```python
from build123d import *

# Parameters (mm, degrees)
BOSS_EXTRUDE1_DEPTH                                 = 40
CUT_EXTRUDE1_DEPTH                                  = 38
BOSS_EXTRUDE2_REACH                                 = 22
SKETCH6_W                                           = 7.999999469
SKETCH6_H                                           = 7.25
BOSS_EXTRUDE3_REACH                                 = 22
SKETCH7_W                                           = 7.999999468
SKETCH7_H                                           = 7.25
SKETCH8_W                                           = 7.999999727
SKETCH8_H                                           = 7.25
BOSS_EXTRUDE4_DEPTH                                 = 19
SKETCH9_W                                           = 7.999999728
SKETCH9_H                                           = 7.25
BOSS_EXTRUDE5_DEPTH                                 = 19
CUT_EXTRUDE4_DEPTH                                  = 0.5
BOSS_EXTRUDE6_DEPTH                                 = 0.5
CUT_EXTRUDE5_START                                  = 1.500005
CUT_EXTRUDE5_DEPTH                                  = 0.5
F_3_CLEARANCE_HOLE1_D                               = 3
F_3_CLEARANCE_HOLE1_DEPTH                           = 0.5
CBORE_FOR_4_BINDING_HEAD_MACHINE_SCREW1_D           = 3.2
CBORE_FOR_4_BINDING_HEAD_MACHINE_SCREW1_DEPTH       = 28
CBORE_FOR_4_BINDING_HEAD_MACHINE_SCREW1_CBORE_D     = 6
CBORE_FOR_4_BINDING_HEAD_MACHINE_SCREW1_CBORE_DEPTH = 19.000000001
CBORE_FOR_4_BINDING_HEAD_MACHINE_SCREW2_D           = 3.2
CBORE_FOR_4_BINDING_HEAD_MACHINE_SCREW2_DEPTH       = 25.25
CBORE_FOR_4_BINDING_HEAD_MACHINE_SCREW2_CBORE_D     = 6
CBORE_FOR_4_BINDING_HEAD_MACHINE_SCREW2_CBORE_DEPTH = 16.250000001
CHAMFER2_SIZE                                       = 0.8
FILLET1_R                                           = 1
FILLET2_R                                           = 4


with BuildPart() as part:
    # Sketch1 → Boss-Extrude1 (new body)
    with BuildSketch(Plane(origin=(19.860869514, 0, 0), x_dir=(0, 0, -1), z_dir=(1, 0, 0))):
        Polygon((0.020116779, -25.909092826), (0.020116779, 25.590907174), (-17.979883221, 25.590907174), (-27.979883221, 15.590907174), (-27.979883221, -25.909092826), align=None)
    extrude(amount=-BOSS_EXTRUDE1_DEPTH)

    # Sketch2 → Cut-Extrude1 (cut)
    with BuildSketch(Plane(origin=(-19.139130486, 0, 0), x_dir=(0, -1, 0), z_dir=(-1, 0, 0))):
        Polygon((-24.590907174, 17.565669658), (-24.590907174, -0.020116779), (24.909092826, -0.020116779), (24.909092826, 26.979883221), (-15.176693611, 26.979883221), align=None)
    extrude(amount=-CUT_EXTRUDE1_DEPTH, mode=Mode.SUBTRACT)

    # Sketch6 → Boss-Extrude2 (add, up to next)
    with BuildSketch(Plane(origin=(0, 0, 7.979883221), x_dir=(-1, 0, 0), z_dir=(0, 0, -1)), mode=Mode.PRIVATE) as boss_extrude2_sk1:
        with Locations((15.139130752, 20.965907174)):
            Rectangle(SKETCH6_W, SKETCH6_H)
    boss_extrude2_tool1 = extrude(boss_extrude2_sk1.sketch, amount=-BOSS_EXTRUDE2_REACH, mode=Mode.PRIVATE) - part.part
    add(boss_extrude2_tool1.solids().sort_by_distance((-15.139131, 20.965907, 7.979883))[0])

    # Sketch7 → Boss-Extrude3 (add, up to next)
    with BuildSketch(Plane(origin=(0, 0, 7.979883221), x_dir=(-1, 0, 0), z_dir=(0, 0, -1)), mode=Mode.PRIVATE) as boss_extrude3_sk1:
        with Locations((-14.86086978, 20.965907174)):
            Rectangle(SKETCH7_W, SKETCH7_H)
    boss_extrude3_tool1 = extrude(boss_extrude3_sk1.sketch, amount=-BOSS_EXTRUDE3_REACH, mode=Mode.PRIVATE) - part.part
    add(boss_extrude3_tool1.solids().sort_by_distance((14.86087, 20.965907, 7.979883))[0])

    # Sketch8 → Boss-Extrude4 (add)
    with BuildSketch(Plane(origin=(0, 0, 26.979883221), x_dir=(-1, 0, 0), z_dir=(0, 0, -1))):
        with Locations((-14.86086965, -21.284092826)):
            Rectangle(SKETCH8_W, SKETCH8_H)
    extrude(amount=BOSS_EXTRUDE4_DEPTH)

    # Sketch9 → Boss-Extrude5 (add)
    with BuildSketch(Plane(origin=(0, 0, 26.979883221), x_dir=(-1, 0, 0), z_dir=(0, 0, -1))):
        with Locations((15.139130622, -21.284092826)):
            Rectangle(SKETCH9_W, SKETCH9_H)
    extrude(amount=BOSS_EXTRUDE5_DEPTH)

    # Sketch10 → Cut-Extrude4 (cut)
    with BuildSketch(Plane.XY.offset(27.979883221)):
        with BuildLine():
            Line((14.150288676, -11.659092827), (2.025933023, 9.340907173))
            ThreePointArc((2.025933023, 9.340907173), (-0.139130487, 10.590907173), (-2.304193997, 9.340907173))
            Line((-2.304193997, 9.340907173), (-14.42854965, -11.659092827))
            ThreePointArc((-14.42854965, -11.659092827), (-14.42854965, -14.159092826), (-12.263486141, -15.409092826))
            Line((-12.263486141, -15.409092826), (11.985225167, -15.409092826))
            ThreePointArc((11.985225167, -15.409092826), (14.150288676, -14.159092826), (14.150288676, -11.659092827))
        make_face()
    extrude(amount=-CUT_EXTRUDE4_DEPTH, mode=Mode.SUBTRACT)

    # Sketch11 → Boss-Extrude6 (add)
    with BuildSketch(Plane.XY.offset(27.479883221)):
        with BuildLine():
            Line((-13.129511542, -12.409092827), (-1.005155889, 8.590907173))
            ThreePointArc((-1.005155889, 8.590907173), (-0.139130485, 9.090907174), (0.72689492, 8.590907173))
            Line((0.72689492, 8.590907173), (12.851250572, -12.409092827))
            ThreePointArc((12.851250572, -12.409092827), (12.851250572, -13.409092827), (11.985225169, -13.909092826))
            Line((11.985225169, -13.909092826), (-12.263486138, -13.909092826))
            ThreePointArc((-12.263486138, -13.909092826), (-13.129511542, -13.409092827), (-13.129511542, -12.409092827))
        make_face()
    extrude(amount=BOSS_EXTRUDE6_DEPTH)

    # Sketch12 → Cut-Extrude5 (cut)
    with BuildSketch(Plane.XY.offset(26.479878344).offset(CUT_EXTRUDE5_START)):
        with BuildLine():
            Line((-1.181805728, -4.919953815), (-1.557388601, 0.642194436))
            add(Edge.make_bspline(
                [(-1.557388601, 0.642194436), (-1.562255195, 0.726894151), (-1.57197876, 0.896126108), (-1.573630596, 1.150381332), (-1.563491274, 1.404367732), (-1.539477279, 1.657492298), (-1.498601615, 1.908446588), (-1.435950641, 2.155034423), (-1.347824447, 2.394209038), (-1.227947002, 2.620066875), (-1.070203444, 2.821498256), (-0.873757735, 2.98640743), (-0.644495445, 3.100925878), (-0.395458992, 3.166647074), (-0.224777297, 3.173588668), (-0.139130486, 3.177071908)],
                knots=[0, 0, 0, 0, 0.076934304, 0.153716488, 0.230489845, 0.307379808, 0.384178278, 0.460861998, 0.537777924, 0.614835636, 0.691825929, 0.768406055, 0.845421183, 0.922433493, 1, 1, 1, 1], degree=3))
            add(Edge.make_bspline(
                [(-0.139130486, 3.177071908), (-0.065510928, 3.174528216), (0.081440904, 3.169450757), (0.298073955, 3.121720242), (0.503386356, 3.037662683), (0.688981961, 2.914531923), (0.846742946, 2.757270627), (0.974882351, 2.575723676), (1.075136008, 2.378059028), (1.151690203, 2.170509138), (1.208454116, 1.957026535), (1.248786563, 1.740308946), (1.275266584, 1.522162803), (1.290343043, 1.303017743), (1.295405911, 1.083047008), (1.292059183, 0.862557831), (1.283440251, 0.71568476), (1.279127629, 0.642194436)],
                knots=[0, 0, 0, 0, 0.06668985, 0.133119456, 0.199920485, 0.266795101, 0.333669142, 0.400733876, 0.467442387, 0.534072191, 0.600968136, 0.667508068, 0.733796294, 0.800115594, 0.866606751, 0.933254524, 1, 1, 1, 1], degree=3))
            Line((1.279127629, 0.642194436), (0.903544756, -4.919953815))
            add(Edge.make_bspline(
                [(0.903544756, -4.919953815), (0.899040298, -4.98465678), (0.890033529, -5.114031861), (0.87358409, -5.307836112), (0.853415093, -5.501287734), (0.828449527, -5.694285405), (0.796710241, -5.88637973), (0.754944033, -6.076605831), (0.700731594, -6.263716972), (0.628895269, -6.444933688), (0.532938656, -6.614900625), (0.405346695, -6.763808252), (0.243240213, -6.874664069), (0.056441287, -6.938986541), (-0.073726294, -6.945537445), (-0.139130486, -6.948829022)],
                knots=[0, 0, 0, 0, 0.076936874, 0.153837066, 0.230708206, 0.307638675, 0.384651809, 0.461589354, 0.538534726, 0.615507305, 0.692327105, 0.769110055, 0.845963233, 0.922602462, 1, 1, 1, 1], degree=3))
            add(Edge.make_bspline(
                [(-0.139130486, -6.948829022), (-0.204192465, -6.945646156), (-0.334523872, -6.939270276), (-0.52166752, -6.874698808), (-0.684560534, -6.763099851), (-0.812386409, -6.613205645), (-0.908338892, -6.442461666), (-0.98006333, -6.260618976), (-1.034024433, -6.073329831), (-1.075624515, -5.883322576), (-1.107062911, -5.691940143), (-1.131842025, -5.499751942), (-1.151924163, -5.306932214), (-1.168322738, -5.113609534), (-1.177310111, -4.984524213), (-1.181805728, -4.919953815)],
                knots=[0, 0, 0, 0, 0.076983897, 0.154213255, 0.231303489, 0.308508561, 0.385703214, 0.462682138, 0.539884122, 0.61667812, 0.693280216, 0.76986989, 0.846510018, 0.923222027, 1, 1, 1, 1], degree=3))
        make_face()
    extrude(amount=-CUT_EXTRUDE5_DEPTH, mode=Mode.SUBTRACT)

    # #3 Clearance Hole1
    with Locations(Plane.XY.offset(27.979883221)):
        with Locations((-0.139130486, -10.159092826)):
            Hole(F_3_CLEARANCE_HOLE1_D / 2, depth=F_3_CLEARANCE_HOLE1_DEPTH)

    # CBORE for #4 Binding Head Machine Screw1
    with Locations(Plane.XY.offset(27.979883221)):
        with Locations((14.860869787, -21.659092826), (-15.139130758, -21.659092826)):
            CounterBoreHole(CBORE_FOR_4_BINDING_HEAD_MACHINE_SCREW1_D / 2, CBORE_FOR_4_BINDING_HEAD_MACHINE_SCREW1_CBORE_D / 2, CBORE_FOR_4_BINDING_HEAD_MACHINE_SCREW1_CBORE_DEPTH, depth=CBORE_FOR_4_BINDING_HEAD_MACHINE_SCREW1_DEPTH)

    # CBORE for #4 Binding Head Machine Screw2
    with Locations(Plane.XY.offset(25.229883221)):
        with Locations((-15.139131017, 21.340907174), (14.860870046, 21.340907174)):
            CounterBoreHole(CBORE_FOR_4_BINDING_HEAD_MACHINE_SCREW2_D / 2, CBORE_FOR_4_BINDING_HEAD_MACHINE_SCREW2_CBORE_D / 2, CBORE_FOR_4_BINDING_HEAD_MACHINE_SCREW2_CBORE_DEPTH, depth=CBORE_FOR_4_BINDING_HEAD_MACHINE_SCREW2_DEPTH)

    # Chamfer2
    chamfer2_edges = [part.edges().sort_by_distance(p)[0] for p in [
        (-20.139130486, 25.590907174, 8.979883221),
        (-20.139130486, -25.909092826, 13.979883221),
        (19.860869514, 25.590907174, 8.979883221),
        (19.860869514, -25.909092826, 13.979883221),
    ]]
    chamfer(chamfer2_edges, length=CHAMFER2_SIZE)

    # Fillet1
    fillet1_edges = [part.edges().sort_by_distance(p)[0] for p in [
        (-11.139131017, 24.590907174, 12.77277644),
        (-19.139130486, 17.340907174, 16.39777644),
        (10.860870046, 24.590907174, 12.77277644),
        (18.860869514, 17.340907174, 16.39777644),
        (10.860869787, -24.909092826, 17.479883221),
        (18.860869514, -17.659092826, 17.479883221),
        (-19.139130486, -17.659092826, 17.479883221),
        (-11.139130758, -24.909092826, 17.479883221),
    ]]
    fillet(fillet1_edges, radius=FILLET1_R)

    # Fillet2
    fillet2_edges = [part.edges().sort_by_distance(p)[0] for p in [
        (-11.139131017, 17.340907174, 16.39777644),
        (10.860870046, 17.340907174, 16.39777644),
        (10.860869787, -17.659092826, 17.479883221),
        (-11.139130758, -17.659092826, 17.479883221),
    ]]
    fillet(fillet2_edges, radius=FILLET2_R)


solid = part.part
```
Can you work these out from the model? Positions are in its coordinate system, mm. A direction names the side the tool comes from. Coordinates: 2 decimals unless noted, no trailing zeros. Loops run counter-clockwise (first coordinate to the right, second up) from the corner with the lowest first, then second, coordinate; pieces in that order, holes last.
1) For pin 1 (6.5 mm diameter, centred on x = 14.5, y = -19.5, fed in from -Z); pin 2 (0.9 mm diameter, centred on x = -1, y = -10.5, fed in from +Z); pin 3 (2 mm diameter, centred on x = 1, z = 21.5, fed in from +Y), each with a flat end and sliding along its axis, tell me the tip position at first contact or that it passes through.
2) Thinking about a two-plate mould opening in Y: for faces 4 (the flat face through (0, 25.591, 9)), 5 (the flat face through (-8.28, -1.01, 27.73)), 6 (the flat face through (0, -7.4, 27.98)), which applies, pulls with the +Y half, pulls with the -Y half, needs draft (parallel to the pull), parting line crosses it, or undercut?
3) Which directions (+Z, -Z, +X, -X, +Y, -Y) give clear straight access to the entire face, cutting with the end or side of a thin tool? Please do faces 1 (the cylindrical face through (-13.75, 18.68, 15.44)), 2 (the flat face through (18.861, 0, 14)), 3 (the cylindrical face through (14, -20.31, 8.47)).
4) Imagine slicing it at B-B on y = 13. List the corners of the cut face in (x, z) for me.
5) Imagine slicing it at C-C on z = 23.25. State how many separate pieces and enclosed holes the cut face has, plus the area to 3 significant figures.
6) Imagine slicing it at A-A on z = 7. List the corners of the cut face in (x, y) for me.
7) I need wall thicknesses on probe 1 along Y at (x, z) = (-15, 12.5); probe 2 along Y at (x, z) = (15, 24.75); probe 3 along X at (y, z) = (-1, 20). Which ranges of each line are inside material? Lowest first, please.
8) Imagine slicing it at D-D on x = 7.5. List the corners of the cut face in (y, z) for me.
Completed:
1. pin 1: stops at z = 7.98
1. pin 2: stops at z = 27.48
1. pin 3: stops at y = 23.07
2. face 4: pulls with the +Y half
2. face 5: undercut
2. face 6: needs draft
3. face 1: +Z
3. face 2: -Z
3. face 3: +Z, -Z
4. outline: (-20.14, -0.02) - (-19.14, -0.02) - (-19.14, 26.98) - (18.86, 26.98) - (18.86, -0.02) - (19.86, -0.02) - (19.86, 27.98) - (-20.14, 27.98) - close
5. separate pieces: 1
5. enclosed holes: 3
5. area: 241 mm2
6. outline: (-20.14, -25.11) - (-19.34, -25.91) - (19.06, -25.91) - (19.86, -25.11) - (19.86, 24.79) - (19.06, 25.59) - (-19.34, 25.59) - (-20.14, 24.79) - close; hole (-19.14, -24.91) - (18.86, -24.91) - (18.86, 24.59) - (-19.14, 24.59) - close
7. probe 1: y = -25.91 to -24.66, -18.66 to -17.66, 17.34 to 18.34, 24.34 to 25.59
7. probe 2: y = -25.91 to -24.66, -18.66 to -17.66, 17.34 to 18.34
7. probe 3: x = -20.14 to -19.14, 18.86 to 19.86
8. outline: (-25.91, -0.02) - (-24.91, -0.02) - (-24.91, 26.98) - (15.18, 26.98) - (24.59, 17.57) - (24.59, -0.02) - (25.59, -0.02) - (25.59, 17.98) - (15.59, 27.98) - (-0.14, 27.98) - (-0.14, 27.48) - (-3.14, 27.48) - (-3.14, 27.98) - (-13.91, 27.98) - (-13.91, 27.48) - (-15.41, 27.48) - (-15.41, 27.98) - (-25.91, 27.98) - close
